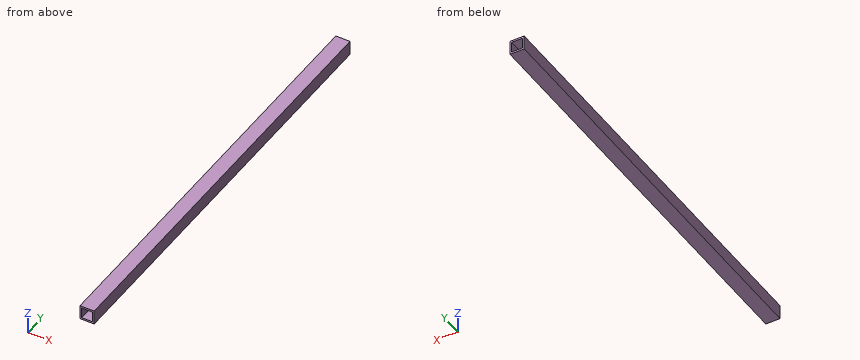
```python
from build123d import *

# Parameters (mm, degrees)
F0_W     = 25.4
F0_H     = 25.4
F1_DEPTH = 762
F2_W     = 19.05
F2_H     = 19.05
F3_DEPTH = 45.72
F4_W     = 19.05
F4_H     = 19.05
F5_DEPTH = 45.72


with BuildPart() as f1:
    # F0 (on Front) → F1 (new body)
    with BuildSketch(Plane.XZ):
        with Locations((-0.477387, 0.30238)):
            Rectangle(F0_W, F0_H)
    extrude(amount=F1_DEPTH)

    # F2 (on face) → F3 (cut)
    with BuildSketch(Plane.XZ.offset(762)):
        with Locations((-0.477387, 0.30238)):
            Rectangle(F2_W, F2_H)
    extrude(amount=-F3_DEPTH, mode=Mode.SUBTRACT)

    # F4 (on face) → F5 (cut)
    with BuildSketch(Plane(origin=(0, 0, 0), x_dir=(-1, 0, 0), z_dir=(0, 1, 0))):
        with Locations((0.477387, 0.30238)):
            Rectangle(F4_W, F4_H)
    extrude(amount=-F5_DEPTH, mode=Mode.SUBTRACT)


solid = f1.part
```
Here's how the part is built. I have some questions about the finished solid (model axes, mm). Give positions to 0.01 mm unless a question says otherwise; leave off trailing zeros. Loops run counter-clockwise (first coordinate to the right, second up) from the corner with the lowest first, then second, coordinate; pieces in that order, holes last. Notation, with made-up numbers: (-40, 41) -> (-27, 41) arc R33 ccw to (-27, 74) -> close; hole circle Ø8 at (55.5, 67.25). An arc over 180 degrees is marked (long way). Use one line per item in the form item = value. Start each with the question number.
1) For P1, Ø2, axis at x = 8.5, z = -9, coming from the +Y side; P2, Ø1.5, axis at x = -7, z = -4, coming from the -Y side; P3, Ø1, axis at x = 1, z = -1.5, coming from the +Y side, each with a flat end and sliding along its axis, tell me the tip position at first contact or that it passes through.
2) Imagine slicing it at B-B (x = 3). Please give me the cut outline in (y, z), then the cut area to 3 significant figures.
3) Imagine slicing it at A-A (z = -1). Please give me the cut outline in (x, y), then the cut area to 3 significant figures.
4) Please list where these lines run through material, in increasing order: line 1 along Z through (x, y) = (3, -34); line 2 along X through (y, z) = (-717.5, 3.5); line 3 along Y through (x, z) = (1.5, 5.5).
Check values:
q1.P1 = 0
q1.P2 = -716.28
q1.P3 = -45.72
q2.outline = (-762, -12.4) -> (0, -12.4) -> (0, -9.22) -> (-45.72, -9.22) -> (-45.72, 9.83) -> (0, 9.83) -> (0, 13) -> (-762, 13) -> (-762, 9.83) -> (-716.28, 9.83) -> (-716.28, -9.22) -> (-762, -9.22) -> close
q2.area = 17,600 mm^2
q3.outline = (-13.18, -762) -> (-10, -762) -> (-10, -716.28) -> (9.05, -716.28) -> (9.05, -762) -> (12.22, -762) -> (12.22, 0) -> (9.05, 0) -> (9.05, -45.72) -> (-10, -45.72) -> (-10, 0) -> (-13.18, 0) -> close
q3.area = 17,600 mm^2
q4.line_1 = -12.4 to -9.22, 9.83 to 13
q4.line_2 = -13.18 to -10, 9.05 to 12.22
q4.line_3 = -716.28 to -45.72
